Source: CAD feature listing. Evaluate the final solid. Frame: model axes, mm. Face numbers are marked on the shaded views. A direction names the side the tool comes from. Give positions to 0.01 mm unless a question says otherwise; leave off trailing zeros. Write each loop counter-clockwise with the first axis right and the second up, starting at its lowest first coordinate (ties: lowest second). Pieces come first, ordered by that corner, then holes. Notation, with made-up numbers: M 70,15.5 L 127,15.5 A17 cw 127,19.5 Z; hole C 21,-21 d1. An arc over 180 degrees is marked long. Return JSON: item names as keys, results as strings.
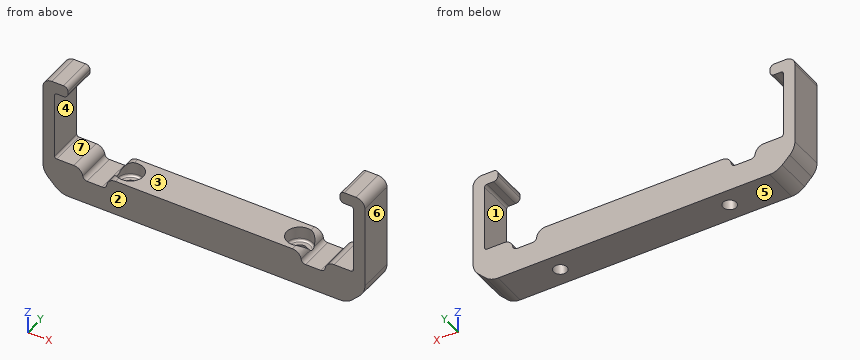
Autodesk Inventor part; units mm, degrees
ref_plane "Work Plane1" through (0, 0, 0) normal (0, 0, 1) x (1, 0, 0)
ref_plane "YZ Plane" through (0, 0, 0) normal (1, 0, 0) x (0, 1, 0)
ref_plane "XZ Plane" through (0, 0, 0) normal (0, 1, 0) x (-1, 0, 0)
ref_plane "Work Plane1" through (0, 0, 0) normal (0, 0, 1) x (1, 0, 0)
sketch "base_sketch" plane through (0, 0, 0) normal (0, 0, 1) x (1, 0, 0)
  circle A0 centre (0, -125.6462) radius 1.5
  circle A1 centre (-38, -125.6462) radius 1.5
  line L0 (14.5, -121.6462) -> (-52.5, -121.6462)
  line L1 (-52.5, -121.6462) -> (-52.5, -129.6462)
  line L2 (-52.5, -129.6462) -> (14.5, -129.6462)
  line L3 (14.5, -129.6462) -> (14.5, -121.6462)
  line L4 (-19, -121.6462) -> (-19, -129.6462) construction
  point P0 (0, 0)
  dimension "d1" = 67
  dimension "d4" = 38
  dimension "d5" = 19
  dimension "d6" = 4
  dimension "d7" = 4
extrude "base" add sketch "base_sketch" along normal blind 8
sketch "holes_bolt_head_sketch" plane through (0, 0, 8) normal (0, 0, 1) x (1, 0, 0)
  circle A0 centre (0, -125.6462) radius 1.5 construction
  circle A1 centre (0, -125.6462) radius 2.9
  circle A2 centre (-38, -125.6462) radius 1.5 construction
  circle A3 centre (-38, -125.6462) radius 2.9
  point P0 (0, 0)
  dimension "d10" = 5.8
  dimension "d11" = 5.8
extrude "holes_bolt_head" cut sketch "holes_bolt_head_sketch" against normal blind 3.2
fillet "bolt_head_fillet" radius 0.5 2 edges at (-40.9, -125.6462, 4.8) (-2.9, -125.6462, 4.8)
sketch "walls_sketch" plane through (-52.5, -129.6462, 0) normal (0, -1, 0) x (1, 0, 0)
  line L0 (0, 0) -> (67, 0)
  line L1 (67, 0) -> (67, 8)
  line L2 (0, 8) -> (67, 8)
  line L3 (0, 0) -> (0, 8)
  line L4 (67, 8) -> (0, 8)
  line L5 (0, 8) -> (0, 23.7)
  line L6 (0, 23.7) -> (3, 23.7)
  line L7 (0, 23.7) -> (3, 23.7) construction
  line L8 (3, 23.7) -> (3, 26.3)
  line L9 (3, 26.3) -> (-2.6, 26.3)
  line L10 (-2.6, 26.3) -> (-2.6, 0)
  line L11 (0, 0) -> (67, 0)
  line L12 (-2.6, 0) -> (0, 0)
  line L13 (0, 0) -> (0, 8)
  line L14 (33.5, 8) -> (33.5, 0) construction
  line L15 (67, 8) -> (67, 23.7)
  line L16 (67, 23.7) -> (64, 23.7)
  line L17 (64, 23.7) -> (64, 26.3)
  line L18 (64, 26.3) -> (69.6, 26.3)
  line L19 (69.6, 26.3) -> (69.6, 0)
  line L20 (69.6, 0) -> (67, 0)
  point P0 (52.5, 0)
  dimension "d15" = 15.7
  dimension "d16" = 3
  dimension "d17" = 0
  dimension "d18" = 2.6
  dimension "d19" = 2.6
extrude "walls" add sketch "walls_sketch" against normal up to surface (8 mm away) contours L12 L10 L9 L8 L6 L5 L3 | L1 L15 L16 L17 L18 L19 L20
fillet "wall_top" radius 2 2 edges at (-55.1, -125.6462, 26.3) (17.1, -125.6462, 26.3)
fillet "wall_tooth" radius 1 4 edges at (-49.5, -125.6462, 26.3) (-49.5, -125.6462, 23.7) (11.5, -125.6462, 23.7) (11.5, -125.6462, 26.3)
chamfer "wall_bottom" distance 4 angle 45 2 edges at (17.1, -125.6462, 0) (-55.1, -125.6462, 0)
fillet "wall_bottom_fillet" radius 4 4 edges at (-55.1, -125.6462, 4) (17.1, -125.6462, 4) (13.1, -125.6462, 0) (-51.1, -125.6462, 0)
fillet "inside" radius 0.5 4 edges at (14.5, -125.6462, 8) (-52.5, -125.6462, 8) (-52.5, -125.6462, 23.7) (14.5, -125.6462, 23.7)
sketch "groove_enclosure_bolt_sketch" plane through (-53.1, -121.6462, 26.3) normal (0, 1, 0) x (1, 0, 0)
  line L0 (67.1, 18.3) -> (1.1, 18.3)
  line L1 (55.9, 18.3) -> (61.3, 18.3)
  line L2 (61.3, 18.3) -> (61.3, 19.9)
  line L3 (60.3, 20.9) -> (56.9, 20.9)
  line L4 (55.9, 19.9) -> (55.9, 18.3)
  line L5 (34.1, 18.3) -> (34.1, 26.3) construction
  line L6 (3.6569, 26.3) -> (64.5431, 26.3)
  arc A0 (56.9, 20.9) -> (55.9, 19.9) centre (56.9, 19.9) ccw
  arc A1 (61.3, 19.9) -> (60.3, 20.9) centre (60.3, 19.9) ccw
  line L7 (12.3, 18.3) -> (6.9, 18.3)
  line L8 (6.9, 18.3) -> (6.9, 19.9)
  line L9 (7.9, 20.9) -> (11.3, 20.9)
  line L10 (12.3, 19.9) -> (12.3, 18.3)
  arc A2 (12.3, 19.9) -> (11.3, 20.9) centre (11.3, 19.9) ccw
  arc A3 (7.9, 20.9) -> (6.9, 19.9) centre (7.9, 19.9) ccw
  point P0 (53.1, 26.3)
  point P1 (61.3, 20.9)
  point P2 (55.9, 20.9)
  point P3 (58.6, 20.9)
  point P4 (6.9, 18.3)
  point P5 (12.3, 18.3)
  dimension "d29" = 66
  dimension "d30" = 33
  dimension "d31" = 49
  dimension "d32" = 5.4
  dimension "d33" = 2.6
  dimension "d34" = 1
extrude "groove_enclosure_bolt" cut sketch "groove_enclosure_bolt_sketch" against normal through all
fillet "groove_enclosure_bolt_rounded" radius 2 6 edges at (8.2, -125.6462, 8) (2.8, -123.2687, 8) (2.8, -128.0237, 8) (-40.8, -123.2687, 8) (-40.8, -128.0237, 8) (-46.2, -125.6462, 8)
equation "\"d5\" = 0.5 * d4"
equation "\"d7\" = d6"
equation "\"d10\" = d11"
equation "\"d30\" = 0.5 * d29"
properties part number "mount_enclosure_coral_dev_board" material "ABS Plastic"
1) Cut plane B-B, the plane z = 10. Return the cut outline in (x, y).
Numbers:
{"outline": "M -55.1,-129.65 L -52.5,-129.65 L -52.5,-121.65 L -55.1,-121.65 Z; M 14.5,-129.65 L 17.1,-129.65 L 17.1,-121.65 L 14.5,-121.65 Z"}
2) Set-up query: the marked faces 1, 2 and 3. Return all of +Z, -Z, +X, -X, +Y, -Y with unobstructed straight access to the full face (end or side cutting, diameter ignored); none if empty.
Numbers:
{"face 1": "+Y, -Y", "face 2": "+Z, -Z, +X, -X, -Y", "face 3": "+Z, +Y, -Y"}
3) Line query: line 1 (Y direction, x = 0, z = 7.2); line 2 (X direction, y = -124.25, z = 18.75); line 3 (X direction, y = -126.5, z = 5.25). Output: solid intervals per line, ascending. Write a range as [from, to].
Numbers:
{"line 1": "y = [-129.65, -128.55], [-122.75, -121.65]", "line 2": "x = [-55.1, -52.5], [14.5, 17.1]", "line 3": "x = [-55.08, -40.77], [-35.23, -2.77], [2.77, 17.08]"}
4) Cut plane C-C, the plane x = -14.5. Return the cut outline in (y, z).
Numbers:
{"outline": "M -129.65,0 L -121.65,0 L -121.65,8 L -129.65,8 Z"}
5) Contact query for flat-ended pins moving along their axis: pin 1 Ø2.5 at (x, y) = (-38, -125.65) entering from -Z; pin 2 Ø3.5 at (x, y) = (0, -125.65) entering from +Z; pin 3 Ø2 at (x, y) = (-5, -126) entering from +Z; pin 4 Ø0.5 at (y, z) = (-127, 25) entering from -X. Output: stop coordinate, or through.
Numbers:
{"pin 1": "passes through", "pin 2": "stops at z = 4.8", "pin 3": "stops at z = 8", "pin 4": "stops at x = -55.05"}
6) Cut plane A-A, the plane x = 0. Return the cut outline in (y, z).
Numbers:
{"outline": "M -129.65,0 L -127.15,0 L -127.15,4.8 L -128.05,4.8 A0.5 cw -128.55,5.3 L -128.55,8 L -129.65,8 Z; M -124.15,0 L -121.65,0 L -121.65,8 L -122.75,8 L -122.75,5.3 A0.5 cw -123.25,4.8 L -124.15,4.8 Z"}
7) Draft query along Z for the marked faces 4, 5, 6 and 7. Return one class per face: released by +Z, released by -Z, zero draft, split by the parting line, or undercut.
Numbers:
{"face 4": "undercut", "face 5": "released by -Z", "face 6": "zero draft", "face 7": "undercut"}
